```python
from build123d import *

# Parameters (mm, degrees)
BOSS_EXTRUDE1_DEPTH = 66.675
SKETCH3_R           = 1.7
CUT_EXTRUDE1_DEPTH  = 77.603742892
SKETCH6_R           = 1.7
CUT_EXTRUDE2_DEPTH  = 77.170890273
FILLET1_R           = 2.54
SKETCH8_W           = 22.86
SKETCH8_H           = 1.27
BOSS_EXTRUDE2_DEPTH = 17.78
CUT_EXTRUDE5_DEPTH  = 17.78
SKETCH13_W          = 7.62
SKETCH13_H          = 1.27
BOSS_EXTRUDE3_DEPTH = 22.86
CUT_EXTRUDE6_DEPTH  = 22.86
SKETCH15_R          = 1.7
CUT_EXTRUDE7_DEPTH  = 43.18
SKETCH16_W          = 3.048
SKETCH16_H          = 33.655
CUT_EXTRUDE8_DEPTH  = 43.18


with BuildPart() as part:
    # Sketch2 → Boss-Extrude1 (new body)
    with BuildSketch(Plane.XY):
        Polygon((0, 0), (-1.27, 0), (-1.27, 26.67), (25.4, 26.67), (25.4, 25.4), (0, 25.4), align=None)
    extrude(amount=BOSS_EXTRUDE1_DEPTH)

    # Sketch3 → Cut-Extrude1 (cut, through all)
    with BuildSketch(Plane.ZY.offset(1.27)):
        with Locations(Location((10.16, 5.08, 0), (0, 0, 270))):
            Circle(SKETCH3_R)
        with Locations((56.515, 5.08)):
            Circle(SKETCH3_R)
    extrude(amount=-CUT_EXTRUDE1_DEPTH, mode=Mode.SUBTRACT)

    # Sketch6 → Cut-Extrude2 (cut, through all)
    with BuildSketch(Plane(origin=(0, 26.67, 0), x_dir=(1, 0, 0), z_dir=(0, 1, 0))):
        with Locations(Location((20.32, -10.16, 0), (0, 0, 270))):
            Circle(SKETCH6_R)
        with Locations(Location((20.32, -56.515, 0), (0, 0, 270))):
            Circle(SKETCH6_R)
    extrude(amount=-CUT_EXTRUDE2_DEPTH, mode=Mode.SUBTRACT)

    # Fillet1
    fillet1_edges = [part.edges().sort_by_distance(p)[0] for p in [
        (25.4, 26.035, 66.675),
        (-0.635, 0, 66.675),
        (25.4, 26.035, 0),
        (-0.635, 0, 0),
    ]]
    fillet(fillet1_edges, radius=FILLET1_R)

    # Sketch8 → Boss-Extrude2 (add)
    with BuildSketch(Plane.XZ.offset(-25.4)):
        with Locations((11.43, 49.53)):
            Rectangle(SKETCH8_W, SKETCH8_H)
        with Locations((11.43, 17.145)):
            Rectangle(SKETCH8_W, SKETCH8_H)
    extrude(amount=BOSS_EXTRUDE2_DEPTH)

    # Sketch12 → Cut-Extrude5 (cut)
    with BuildSketch(Plane.XZ.offset(-25.4)):
        Polygon((0, 50.165), (22.86, 50.165), (22.86, 48.895), (0, 48.895), (0, 17.78), (22.86, 17.78), (22.86, 16.51), (0, 16.51), (0, 0), (31.875752577, 0), (31.875752577, 66.675), (0, 66.675), align=None)
    extrude(amount=-CUT_EXTRUDE5_DEPTH, mode=Mode.SUBTRACT)

    # Sketch13 → Boss-Extrude3 (add)
    with BuildSketch(Plane(origin=(0, 0, 0), x_dir=(0, 0, -1), z_dir=(1, 0, 0))):
        with Locations((-45.085, 10.795)):
            Rectangle(SKETCH13_W, SKETCH13_H)
        with Locations((-21.59, 10.795)):
            Rectangle(SKETCH13_W, SKETCH13_H)
        with Locations((-21.59, 23.495)):
            Rectangle(SKETCH13_W, SKETCH13_H)
        with Locations((-45.085, 23.495)):
            Rectangle(SKETCH13_W, SKETCH13_H)
    extrude(amount=BOSS_EXTRUDE3_DEPTH)

    # Sketch14 → Cut-Extrude6 (cut)
    with BuildSketch(Plane.XZ.offset(-10.16)):
        Polygon((0, 41.275), (22.86, 41.275), (22.86, 48.895), align=None)
        Polygon((22.86, 25.4), (22.86, 17.78), (0, 25.4), align=None)
    extrude(amount=-CUT_EXTRUDE6_DEPTH, mode=Mode.SUBTRACT)

    # Sketch15 → Cut-Extrude7 (cut)
    with BuildSketch(Plane.XY.offset(50.165)):
        with Locations((15.978351822, 17.145)):
            Circle(SKETCH15_R)
    extrude(amount=-CUT_EXTRUDE7_DEPTH, mode=Mode.SUBTRACT)

    # Sketch16 → Cut-Extrude8 (cut)
    with BuildSketch(Plane(origin=(0, 26.67, 0), x_dir=(1, 0, 0), z_dir=(0, 1, 0))):
        with Locations((21.336, -33.3375)):
            Rectangle(SKETCH16_W, SKETCH16_H)
    extrude(amount=-CUT_EXTRUDE8_DEPTH, mode=Mode.SUBTRACT)


solid = part.part
```
For this review, take the finished solid that the model builds, in its own axes (mm). A direction names the side the tool comes from. Coordinates: 2 decimals unless noted, no trailing zeros. Write each loop counter-clockwise with the first axis right and the second up, starting at its lowest first coordinate (ties: lowest second). Pieces come first, ordered by that corner, then holes. Notation, with made-up numbers: (-28, 11) -> (-18, 11) arc R15 ccw to (-18, 23) -> close; hole circle Ø7 at (84, 17). An arc over 180 degrees is marked (long way). Put each result on its own line as item: value.
Q1. Take a section at B-B, the plane y = 5.08. State the section outline as (x, z) points (3 decimals).
From the geometry:
outline: (-1.27, 0) -> (0, 0) -> (0, 8.46) -> (-1.27, 8.46) -> close; (-1.27, 11.86) -> (0, 11.86) -> (0, 54.815) -> (-1.27, 54.815) -> close; (-1.27, 58.215) -> (0, 58.215) -> (0, 66.675) -> (-1.27, 66.675) -> close
Q2. Wall thickness on L1, parallel to Y at x = 6.75, z = 21; L2, parallel to Z at x = 3.75, y = 8 (3 decimals); L3, parallel to X at y = 1.75, z = 62: over which ranges is each line inside the solid? List them lowest first.
From the geometry:
L1: y = 10.16 to 11.43, 22.86 to 24.13
L2: z = 16.51 to 17.78, 48.895 to 50.165
L3: x = -1.27 to 0
Q3. Take a section at D-D, the plane x = 17. Count the separate pieces of the cut face and the enclosed holes in it, then the cut area to 3 significant figures.
From the geometry:
separate pieces: 4
enclosed holes: 0
area: 51.4 mm2
Q4. The part is to be moulded in two halves that separate along Y. For faces 1 (the cylindrical face through (-0.644, 0.724, 65.911)), 2 (the flat face through (10.04, 23.49, 44.62)), 3 (the flat face through (8, 24.13, 46)), 4 (the flat face through (8, 22.86, 46)), say which applies: +Y half, -Y half, draft (parallel to the pull), parting line (faces both ways), or undercut.
From the geometry:
face 1: -Y half
face 2: draft
face 3: +Y half
face 4: undercut
Q5. Tool access review of faces 5 (the flat face through (10, 9, 48.895)), 6 (the flat face through (8, 22.86, 21)), 7 (the flat face through (10, 25, 48.895)), 8 (the flat face through (10, 7.62, 17)): name each direction out of +Z, -Z, +X, -X, +Y, -Y from which nothing blocks a thin tool from reaching the whole face with its end or side.
From the geometry:
face 5: +X, -Y
face 6: +X
face 7: +X, +Y
face 8: +Z, -Z, +X, -Y
Q6. Clearance check with flat-ended pins moving along their axes: pin 1 Ø1.5 at (x, z) = (17, 22.5) entering from -Y; pin 2 Ø4 at (x, z) = (13, 45.5) entering from -Y; pin 3 Ø4 at (x, y) = (12.5, 12.5) entering from -Z; pin 4 Ø12 at (x, y) = (4, 19) entering from -Z. State where each tip first meets the part, or that it passes through.
From the geometry:
pin 1: passes through
pin 2: stops at y = 10.16
pin 3: stops at z = 16.51
pin 4: stops at z = 0
Q7. Take a section at A-A, the plane z = 10.16. State the section outline as (x, y) points.
From the geometry:
outline: (-1.27, 0) -> (0, 0) -> (0, 3.38) -> (-1.27, 3.38) -> close; (-1.27, 6.78) -> (0, 6.78) -> (0, 26.67) -> (-1.27, 26.67) -> close
Q8. Take a section at C-C, the plane x = 4.5. State the section outline as (y, z) points (3 decimals), then the cut area to 3 significant figures.
From the geometry:
outline: (7.62, 16.51) -> (26.67, 16.51) -> (26.67, 17.78) -> (24.13, 17.78) -> (24.13, 23.9) -> (22.86, 23.9) -> (22.86, 17.78) -> (11.43, 17.78) -> (11.43, 23.9) -> (10.16, 23.9) -> (10.16, 17.78) -> (7.62, 17.78) -> close; (7.62, 48.895) -> (10.16, 48.895) -> (10.16, 42.775) -> (11.43, 42.775) -> (11.43, 48.895) -> (22.86, 48.895) -> (22.86, 42.775) -> (24.13, 42.775) -> (24.13, 48.895) -> (26.67, 48.895) -> (26.67, 50.165) -> (7.62, 50.165) -> close
area: 79.5 mm2
